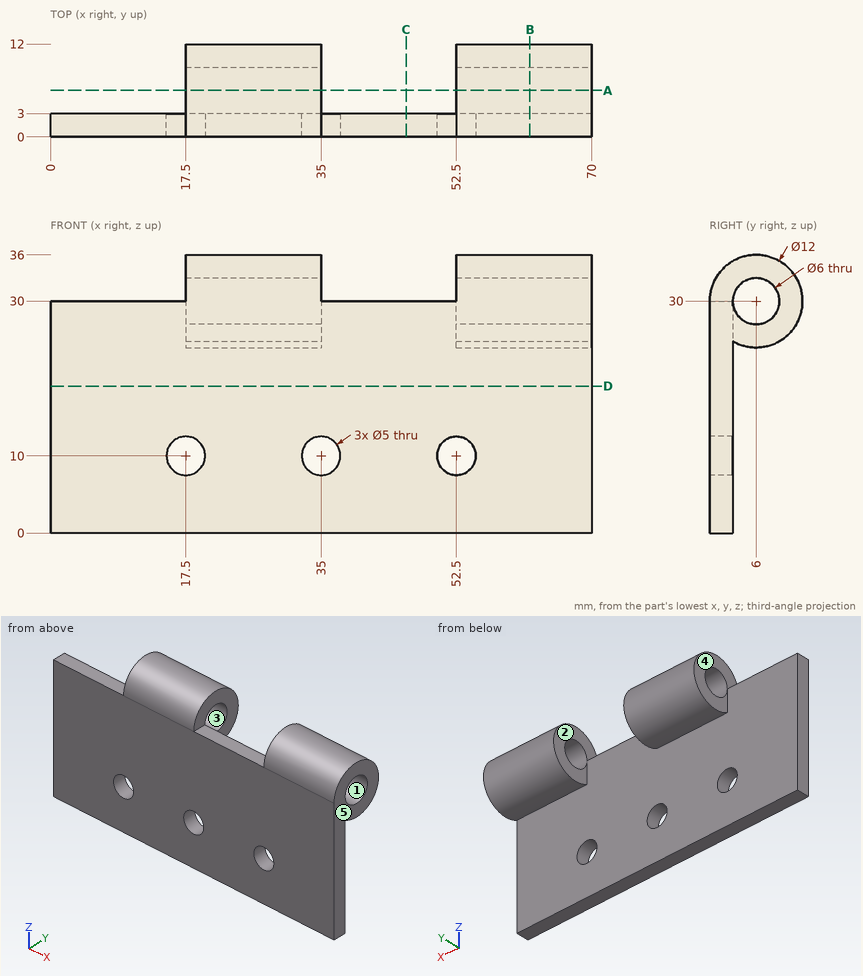
Can you work these out from the drawing? Everything is in mm from the part's minimum corner. A direction names the side the tool comes from. Coordinates: 2 decimals unless noted, no trailing zeros. Write each loop counter-clockwise with the first axis right and the second up, starting at its lowest first coordinate (ties: lowest second). Pieces come first, ordered by that corner, then holes. Notation, with made-up numbers: (-6.75, 41.25) - (18.25, 41.25) arc R22 cw to (18.25, 64.25) - close; hole circle Ø1 at (53.5, 51.5). An arc over 180 degrees is marked (long way). One line per item, written item: value.
1) Suppose I cut it at C-C on x = 46. Write out the boundary of the cut face in (y, z), and give its area (3 significant figures).
Model answer:
outline: (0, 0) - (3, 0) - (3, 30) - (0, 30) - close
area: 90.0 mm²
2) I'm going to push flat-ended pins straight in: P1, Ø3.5, axis at y = 6, z = 30, coming from the +X side; P2, Ø5, axis at x = 28.5, z = 6.5, coming from the +Y side; P3, Ø4, axis at x = 33.5, y = 8.5, coming from the -Z side; P4, Ø3.5, axis at x = 41, y = 1, coming from the +Z side. Where does each tip first touch, or does it pass through?
Model answer:
P1: passes through
P2: stops at y = 3
P3: stops at z = 24.02
P4: stops at z = 30
3) Suppose I cut it at A-A on y = 6. Write out the boundary of the cut face in (x, z).
Model answer:
outline: (17.5, 24) - (35, 24) - (35, 27) - (17.5, 27) - close; (17.5, 33) - (35, 33) - (35, 36) - (17.5, 36) - close; (52.5, 24) - (70, 24) - (70, 27) - (52.5, 27) - close; (52.5, 33) - (70, 33) - (70, 36) - (52.5, 36) - close
4) Suppose I cut it at D-D on z = 19. Write out the boundary of the cut face in (x, y), and give its area (3 significant figures).
Model answer:
outline: (0, 0) - (70, 0) - (70, 3) - (0, 3) - close
area: 210 mm²
5) On a 3-axis mill with a long thin cutter (end or side, diameter ignored), from which of +Z, -Z, +X, -X, +Y, -Y can I reach the whole of each face in a straight line? I mean the marked faces 4 and 5. Say none if no direction works.
Model answer:
face 4: +Z, -X, +Y
face 5: +Z, -Z, +X, +Y, -Y
6) Suppose I cut it at B-B on x = 62. Write out the boundary of the cut face in (y, z).
Model answer:
outline: (0, 0) - (3, 0) - (3, 24.8) arc R6 ccw (long way) to (0, 30) - close; hole circle Ø6 at (6, 30)
7) I need wall thicknesses on line 1 along X through (y, z) = (2.35, 10); line 2 along Z through (x, y) = (62.5, 6); line 3 along Y through (x, z) = (27, 30). Which ranges of each line are inside material? Lowest first, please.
Model answer:
line 1: x = 0 to 15, 20 to 32.5, 37.5 to 50, 55 to 70
line 2: z = 24 to 27, 33 to 36
line 3: y = 0 to 3, 9 to 12
8) We'd pull the mould along Z, two halves only. Please class the marked faces 1, 2 and 3: pulls with the +Z half, pulls with the -Z half, needs draft (parallel to the pull), parting line crosses it, or undercut.
Model answer:
face 1: undercut
face 2: needs draft
face 3: undercut
